Design review of the part shown in the three views and the two pictorial views. Dimensions are in mm from the part's minimum x, y and z. A direction names the side the tool comes from. Give positions to 0.01 mm unless a question says otherwise; leave off trailing zeros. Order: outer loops, then holes, each group sorted by start corner. A loop starts at its lowest first (then second) coordinate and runs counter-clockwise, first axis right, second up.
Item 1: Consider section C-C (y = 119). Give the boundary of the cut face in (x, z).
Item 2: Machinability: for the marked faces 1 and 2, which of the approach directions +Z, -Z, +X, -X, +Y, -Y give a long, thin tool a straight path to every point of the face, cutting with its end or side? Answer none if there is none.
Item 3: For P1, Ø25, axis at x = 81.5, z = 33.5, coming from the +Y side; P2, Ø6, axis at x = 88.5, y = 102, coming from the +Z side, all flat-tipped, find the tip position at first contact; note any pin that passes through.
Item 4: Consider section B-B (x = 85). Give the boundary of the cut face in (y, z).
Item 5: Consider section A-A (x = 25). Give the boundary of the cut face in (y, z), plus the area to 3 significant figures.
Item 6: For probe 1 along X at (y, z) = (4, 35); probe 2 along Z at (x, y) = (25, 5.5); probe 3 along Z at (x, y) = (102, 32.5), list the stretches that pass through material, from the lowest coordinate up.
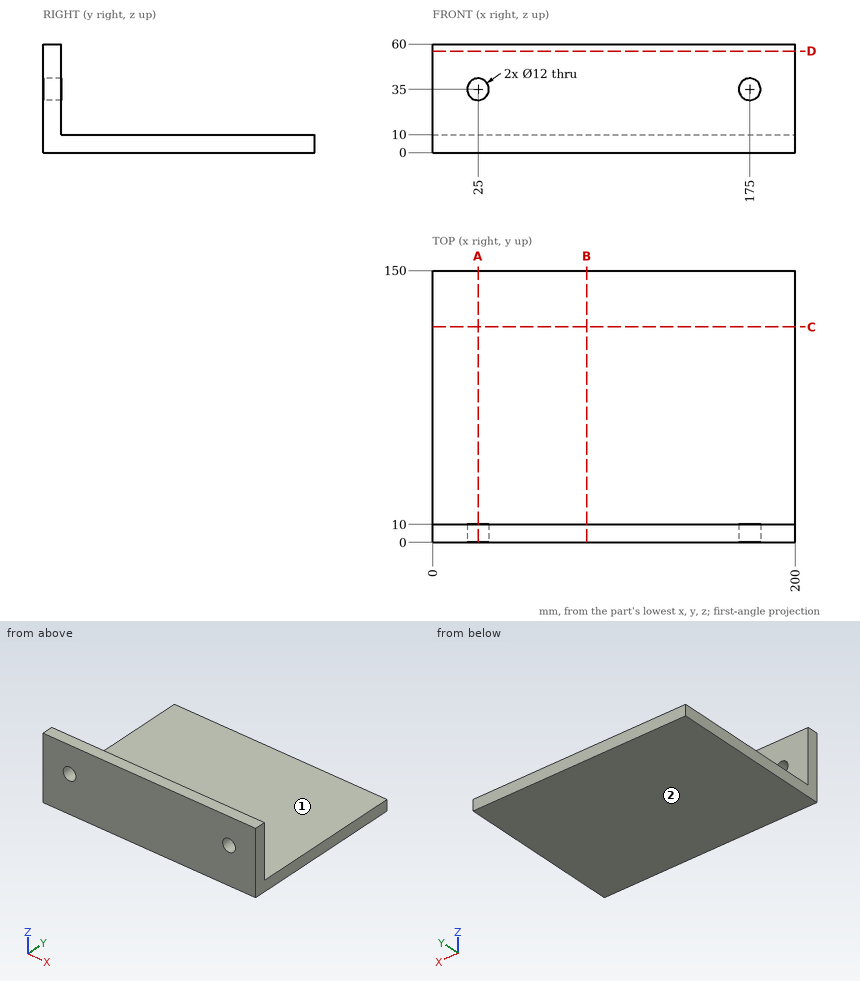
Resolved:
1. outline: (0, 0) - (200, 0) - (200, 10) - (0, 10) - close
2. face 1: +Z, +X, -X, +Y
2. face 2: -Z, +X, -X, +Y, -Y
3. P1: stops at y = 10
3. P2: stops at z = 10
4. outline: (0, 0) - (150, 0) - (150, 10) - (10, 10) - (10, 60) - (0, 60) - close
5. outline: (0, 0) - (150, 0) - (150, 10) - (10, 10) - (10, 29) - (0, 29) - close; (0, 41) - (10, 41) - (10, 60) - (0, 60) - close
5. area: 1,880 mm2
6. probe 1: x = 0 to 19, 31 to 169, 181 to 200
6. probe 2: z = 0 to 29, 41 to 60
6. probe 3: z = 0 to 10
